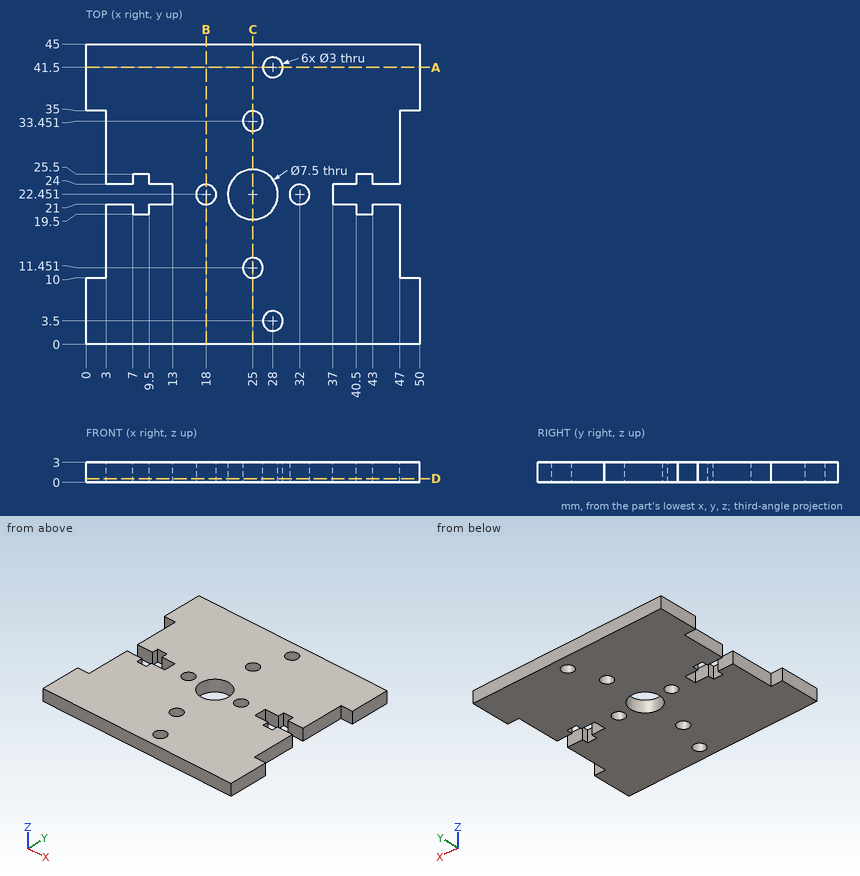
Design review of the part shown in the three views and the two pictorial views. Dimensions are in mm from the part's minimum x, y and z. Round coordinates to 2 decimals unless told otherwise and drop trailing zeros. Write each loop counter-clockwise with the first axis right and the second up, starting at its lowest first coordinate (ties: lowest second). Pieces come first, ordered by that corner, then holes. Notation, with made-up numbers: (-37, 74) - (-3, 74) arc R10 cw to (-3, 78) - close; hole circle Ø11 at (60, 42). An arc over 180 degrees is marked (long way). Answer as CSV lines item,"result". Start each with the question number.
(1) Add section B-B, the plane x = 18. State the section outline as (y, z) points, plus the area to 3 significant figures.
(2) For line 1 (Y direction, x = 32, z = 1.35); line 2 (Y direction, x = 25, z = 1); line 3 (X direction, y = 41.5, z = 1.75), list the stretches that pass through material, from the lowest coordinate up.
(3) For pin 1 (0.8 mm diameter, centred on y = 24.5, z = 1, fed in from -X); pin 2 (1.6 mm diameter, centred on y = 20.5, z = 2, fed in from +X), all flat-tipped, find the tip position at first contact; note any pin that passes through.
(4) Add section D-D, the plane z = 0.55. State how many separate pieces and enclosed holes the cut face has, plus the area to 3 significant figures.
(5) Add section C-C, the plane x = 25. State the section outline as (y, z) points, plus the area to 3 significant figures.
(6) Add section A-A, the plane y = 41.5. State the section outline as (x, z) points, plus the area to 3 significant figures.
From the geometry:
1,outline,"(0, 0) - (20.95, 0) - (20.95, 3) - (0, 3) - close; (23.95, 0) - (45, 0) - (45, 3) - (23.95, 3) - close"
1,area,"126 mm²"
2,line 1,"y = 0 to 20.95, 23.95 to 45"
2,line 2,"y = 0 to 9.95, 12.95 to 18.7, 26.2 to 31.95, 34.95 to 45"
2,line 3,"x = 0 to 26.5, 29.5 to 50"
3,pin 1,"stops at x = 3"
3,pin 2,"stops at x = 47"
4,separate pieces,"1"
4,enclosed holes,"7"
4,area,"1,940 mm²"
5,outline,"(0, 0) - (9.95, 0) - (9.95, 3) - (0, 3) - close; (12.95, 0) - (18.7, 0) - (18.7, 3) - (12.95, 3) - close; (26.2, 0) - (31.95, 0) - (31.95, 3) - (26.2, 3) - close; (34.95, 0) - (45, 0) - (45, 3) - (34.95, 3) - close"
5,area,"94.5 mm²"
6,outline,"(0, 0) - (26.5, 0) - (26.5, 3) - (0, 3) - close; (29.5, 0) - (50, 0) - (50, 3) - (29.5, 3) - close"
6,area,"141 mm²"
